Here's how the part is built. I have some questions about the finished solid (model axes, mm). Face numbers are marked on the shaded views. A direction names the side the tool comes from. Round coordinates to 2 decimals unless told otherwise and drop trailing zeros. Write each loop counter-clockwise with the first axis right and the second up, starting at its lowest first coordinate (ties: lowest second). Pieces come first, ordered by that corner, then holes. Notation, with made-up numbers: (-12.75, 60) - (-1.75, 60) arc R14 ccw to (-1.75, 74) - close; hole circle Ø3 at (-29, 78). An arc over 180 degrees is marked (long way). One line per question, with ' | ' between items. Start each with the question number.
(1) Imagine slicing it at C-C (y = -68). Write out the boundary of the cut face in (x, z), plus the area to 3 significant figures.
(2) For the marked faces 5 and 6, which set-ups out of +Z, -Z, +X, -X, +Y, -Y let a thin tool reach every point of the face, with its end or its side?
(3) Will these pins go through, and if not, where does the flat tip stop? pin 1 (4 mm diameter, centred on x = -131.5, y = -21, fed in from -Z); pin 2 (6 mm diameter, centred on x = -26.5, y = 55.5, fed in from -Z); pin 3 (4 mm diameter, centred on y = 62.5, z = -51.5, fed in from +X).
(4) Thinking about a two-plate mould opening in Y: for the marked faces 1, 2, 3 and 4, which applies, pulls with the +Y half, pulls with the -Y half, needs draft (parallel to the pull), parting line crosses it, or undercut?
(5) Imagine slicing it at B-B (x = 21). Write out the boundary of the cut face in (y, z).
(6) If I drill on L1, parallel to Y at x = -97, z = -11; L2, parallel to Z at x = -46, y = 49.5, over which ranges is the centre line in solid material (lowest first)?
(7) Imagine slicing it at A-A (z = -39). Write out the boundary of the cut face in (x, y), plus the area to 3 significant figures.
from build123d import *

# Parameters (mm, degrees)
SKETCH_1_W               = 270
SKETCH_1_H               = 170
EXTRUDE_1_DEPTH          = 10
SKETCH_3_W               = 270
SKETCH_3_H               = 170
SKETCH_3_W_2             = 260
SKETCH_3_H_2             = 160
EXTRUDE_2_DEPTH          = 70
CUT_EXTRUDE_1_DEPTH      = 292.590466236
CUT_EXTRUDE_1_DEPTH_BACK = 292.590466236
SKETCH_4_W               = 60
SKETCH_4_H               = 130


with BuildPart() as part:
    # 草图1 → 凸台-拉伸1 (new body)
    with BuildSketch(Plane.XY):
        Rectangle(SKETCH_1_W, SKETCH_1_H)
    extrude(amount=EXTRUDE_1_DEPTH)

    # 草图3 → 凸台-拉伸2 (add)
    with BuildSketch(Plane(origin=(0, 0, 0), x_dir=(-1, 0, 0), z_dir=(0, 0, -1))):
        Rectangle(SKETCH_3_W, SKETCH_3_H)
        Rectangle(SKETCH_3_W_2, SKETCH_3_H_2, mode=Mode.SUBTRACT)
    extrude(amount=EXTRUDE_2_DEPTH)

    # 草图4 → 切除-拉伸1 (cut, two sides: drawn at the far end of the back side and taken through both)
    with BuildSketch(Plane(origin=(135, 0, 0), x_dir=(0, 0, -1), z_dir=(1, 0, 0)).offset(-CUT_EXTRUDE_1_DEPTH_BACK)):
        with Locations((40, 0)):
            Rectangle(SKETCH_4_W, SKETCH_4_H)
    extrude(amount=CUT_EXTRUDE_1_DEPTH + CUT_EXTRUDE_1_DEPTH_BACK, mode=Mode.SUBTRACT)


solid = part.part
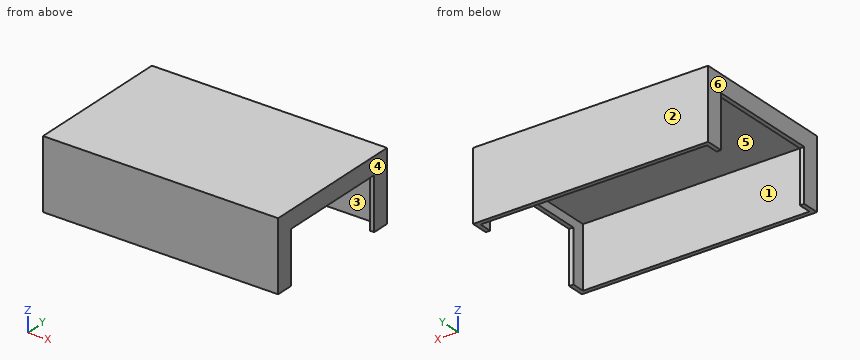
Check sheet entries:
1) outline: (-135, -70) - (-130, -70) - (-130, 0) - (130, 0) - (130, -70) - (135, -70) - (135, 10) - (-135, 10) - close | area: 3,400 mm^2
2) face 5: -Z | face 6: +Z, -Z, -X, +Y, -Y
3) pin 1: z = -10 | pin 2: z = 0 | pin 3: through
4) face 1: undercut | face 2: pulls with the +Y half | face 3: undercut | face 4: needs draft
5) outline: (-85, -70) - (-80, -70) - (-80, 0) - (80, 0) - (80, -70) - (85, -70) - (85, 10) - (-85, 10) - close
6) L1: -85 to -80, 80 to 85 | L2: 0 to 10
7) outline: (-135, -85) - (135, -85) - (135, -65) - (130, -65) - (130, -80) - (-130, -80) - (-130, -65) - (-135, -65) - close; (-135, 65) - (-130, 65) - (-130, 80) - (130, 80) - (130, 65) - (135, 65) - (135, 85) - (-135, 85) - close | area: 3,000 mm^2
